from build123d import *

# Parameters (mm, degrees)
F1_DEPTH = 20
F2_T     = -1
F3_R     = 3
F4_DEPTH = 1.001
F5_R     = 3
F6_DEPTH = 31.001


with BuildPart() as f1:
    # F0 (on Front) → F1 (new body)
    with BuildSketch(Plane.XZ):
        Polygon((70, 30), (70, 40), (48, 40), (12, 10), (-10, 10), (-10, 0), (12, 0), (48, 30), align=None)
    extrude(amount=-F1_DEPTH)

    # F2
    f2_openings = [f1.faces().sort_by_distance(p)[0] for p in [
        (59, 10, 40),
        (30, 10, 25),
        (1, 10, 10),
        (70, 10, 35),
        (-10, 10, 5),
    ]]
    offset(amount=F2_T, openings=f2_openings, kind=Kind.INTERSECTION)

    # F3 (on face) → F4 (cut, through all)
    with BuildSketch(Plane.XY.offset(1)):
        with Locations((0, 10)):
            Circle(F3_R)
    extrude(amount=-F4_DEPTH, mode=Mode.SUBTRACT)

    # F5 (on face) → F6 (cut, through all)
    with BuildSketch(Plane.XY.offset(31)):
        with Locations((60, 10)):
            Circle(F5_R)
    extrude(amount=-F6_DEPTH, mode=Mode.SUBTRACT)


solid = f1.part
Verification items for the finished model (mm, model axes). A direction names the side the tool comes from. Coordinates: 2 decimals unless noted, no trailing zeros. Order: outer loops, then holes, each group sorted by start corner. A loop starts at its lowest first (then second) coordinate and runs counter-clockwise, first axis right, second up. Notation, with made-up numbers: (-14, 61.5) -> (28, 61.5) arc R23 cw to (28, 93.5) -> close; hole circle Ø11 at (39.25, 53). An arc over 180 degrees is marked (long way). Put each result on its own line as item: value. Start each with the question number.
1. Access from +Z, -Z, +X, -X, +Y, -Y to the whole of each face (thin tool, end or side, straight path). Record for faces 1 (the flat face through (3, 12, 1)), 2 (the flat face through (56, 10, 31)), 3 (the flat face through (30, 20, 22)), 4 (the flat face through (56, 10, 30)), 5 (the flat face through (30.25, 0.49, 25.21)).
2. Material ranges on L1, parallel to Y at x = 60, z = 30.5; L2, parallel to Y at x = 56, z = 38; L3, parallel to Z at x = -2, y = 16.5, recorded low to high. Write a range as [from, to].
3. Cross-section at A-A, the plane x = 0. Record the boundary of the cut face in (y, z), then the cut area to 3 significant figures.
4. Cross-section at D-D, the plane y = 14.75. Record the boundary of the cut face in (x, z), then the cut area to 3 significant figures.
5. Mould release check, pull along X, two halves, no side actions. Record for faces 6 (the flat face through (30, 0, 22)), 7 (the flat face through (-10, 10.7, 0.6)), 8 (the cylindrical face through (-3, 10.1, 0.5)): released by +X, released by -X, zero draft, split by the parting line, or undercut.
6. Cross-section at C-C, the plane x = 58.5. Record the boundary of the cut face in (y, z), then the cut area to 3 significant figures.
7. Go/stop test with flat-tipped pins: pin 1 Ø1.1 at (x, y) = (-0.5, 19.5) entering from +Z; pin 2 Ø1.5 at (y, z) = (16.5, 26.5) entering from +X; pin 3 Ø12 at (y, z) = (11.5, 13.5) entering from -X. Record where each tip stops, or that it passes through.
8. Cross-section at B-B, the plane y = 10. Record the boundary of the cut face in (x, z), then the cut area to 3 significant figures.
Computed:
1. face 1: +Z, -X
1. face 2: +Z, +X, -X
1. face 3: +Z, -Z, +X, -X, +Y
1. face 4: -Z, +X, +Y, -Y
1. face 5: +Z, -X, +Y, -Y
2. L1: [0, 7], [13, 20]
2. L2: [0, 1], [19, 20]
2. L3: [0, 1]
3. outline: (0, 0) -> (7, 0) -> (7, 1) -> (1, 1) -> (1, 10) -> (0, 10) -> close; (13, 0) -> (20, 0) -> (20, 10) -> (19, 10) -> (19, 1) -> (13, 1) -> close
3. area: 32.0 mm2
4. outline: (-10, 0) -> (12, 0) -> (48, 30) -> (70, 30) -> (70, 31) -> (47.64, 31) -> (11.64, 1) -> (-10, 1) -> close
4. area: 90.9 mm2
5. face 6: zero draft
5. face 7: released by -X
5. face 8: undercut
6. outline: (0, 30) -> (7.4, 30) -> (7.4, 31) -> (1, 31) -> (1, 40) -> (0, 40) -> close; (12.6, 30) -> (20, 30) -> (20, 40) -> (19, 40) -> (19, 31) -> (12.6, 31) -> close
6. area: 32.8 mm2
7. pin 1: z = 10
7. pin 2: x = 44.7
7. pin 3: x = 19.44
8. outline: (-10, 0) -> (-3, 0) -> (-3, 1) -> (-10, 1) -> close; (3, 0) -> (12, 0) -> (48, 30) -> (57, 30) -> (57, 31) -> (47.64, 31) -> (11.64, 1) -> (3, 1) -> close; (63, 30) -> (70, 30) -> (70, 31) -> (63, 31) -> close
8. area: 78.9 mm2
